Can you work these out from the model? Positions are in its coordinate system, mm. A direction names the side the tool comes from. Round coordinates to 2 decimals unless told otherwise and drop trailing zeros. Loops run counter-clockwise (first coordinate to the right, second up) from the corner with the lowest first, then second, coordinate; pieces in that order, holes last.
from build123d import *

# Parameters (mm, degrees)
ESBO_O1_R                = 6.5
RESSALTO_EXTRUS_O1_DEPTH = 15
RESSALTO_EXTRUS_O2_DEPTH = 35
CORTE_EXTRUS_O1_REACH    = 88.344


with BuildPart() as part:
    # Esboço1 → Ressalto-extrusão1 (new body)
    with BuildSketch(Plane.XY):
        Polygon((-31.616849906, 46.570948478), (-50.373293376, -23.429051522), (-76.616849906, -23.429051522), (-76.616849906, 16.570948478), (-111.616849906, 16.570948478), (-111.616849906, 46.570948478), align=None)
        with Locations((-96.616849906, 31.570948478)):
            Circle(ESBO_O1_R, mode=Mode.SUBTRACT)
    extrude(amount=RESSALTO_EXTRUS_O1_DEPTH)

    # Esboço2 → Ressalto-extrusão2 (add)
    with BuildSketch(Plane(origin=(0, 0, 0), x_dir=(-1, 0, 0), z_dir=(0, 0, -1))):
        Polygon((58.655502819, -23.429051522), (39.899059349, 46.570948478), (31.616849906, 46.570948478), (50.373293376, -23.429051522), align=None)
    extrude(amount=RESSALTO_EXTRUS_O2_DEPTH)

    # Esboço3 → Corte-extrusão1 (cut, up to next)
    with BuildSketch(Plane(origin=(-41.141659675, 11.023874485, 0), x_dir=(0, 0, -1), z_dir=(0.9659258262890673, -0.25881904510252474, 0)), mode=Mode.PRIVATE) as corte_extrus_o1_sk1:
        with BuildLine():
            Line((13, 21.801038988), (13, -16.198961012))
            ThreePointArc((13, -16.198961012), (19, -22.198961012), (25, -16.198961012))
            Line((25, -16.198961012), (25, 21.801038988))
            ThreePointArc((25, 21.801038988), (19, 27.801038988), (13, 21.801038988))
        make_face()
    corte_extrus_o1_tool1 = extrude(corte_extrus_o1_sk1.sketch, amount=-CORTE_EXTRUS_O1_REACH, mode=Mode.PRIVATE) & part.part
    add(corte_extrus_o1_tool1.solids().sort_by_distance((-40.416697, 13.72947, -19))[0], mode=Mode.SUBTRACT)


solid = part.part
(1) Will these pins go through, and if not, where does the flat tip stop? P1, Ø1, axis at x = -55.5, y = 18.5, coming from the -Z side; P2, Ø6, axis at y = -15.5, z = -12.5, coming from the -X side; P3, Ø3, axis at y = 29, z = -4, coming from the -X side.
Worked answers:
P1: stops at z = 0
P2: stops at x = -57.33
P3: stops at x = -45.01
(2) If we section it at A-A, the plane z = -16.5: List the corners of the cut face in (x, y) for me.
Worked answers:
outline: (-58.66, -23.43) - (-50.37, -23.43) - (-46.75, -9.89) - (-54.47, -7.82) - close; (-41.81, 39.42) - (-34.09, 37.35) - (-31.62, 46.57) - (-39.9, 46.57) - close
(3) If we section it at D-D, the plane y = 8.5: List the corners of the cut face in (x, z) for me.
Worked answers:
outline: (-76.62, 0) - (-50.1, 0) - (-50.1, -13) - (-41.82, -13) - (-41.82, 15) - (-76.62, 15) - close; (-50.1, -35) - (-41.82, -35) - (-41.82, -25) - (-50.1, -25) - close
(4) If we mould it in two halves opening along Z, with no side actions, what happens to faces 4 (the flat face through (-44, 14, -25)), 5 (the flat face through (-63, 46.571, 1)), 6 (the flat face through (-43, 12, -35))? For each: released by +Z, released by -Z, zero draft, split by the parting line, or undercut.
Worked answers:
face 4: undercut
face 5: zero draft
face 6: released by -Z
(5) If we section it at B-B, the plane y = 23.5: List the corners of the cut face in (x, z) for me, then the cut area to 3 significant figures.
Worked answers:
outline: (-111.62, 0) - (-46.08, 0) - (-46.08, -13) - (-37.8, -13) - (-37.8, 15) - (-111.62, 15) - close; (-46.08, -35) - (-37.8, -35) - (-37.8, -25) - (-46.08, -25) - close
area: 1,300 mm2
(6) If we section it at C-C, the plane x = -102: List the corners of the cut face in (y, z) for me.
Worked answers:
outline: (16.57, 0) - (27.93, 0) - (27.93, 15) - (16.57, 15) - close; (35.21, 0) - (46.57, 0) - (46.57, 15) - (35.21, 15) - close
(7) If I drill on line 1 (Z direction, x = -47, y = 11.5); line 2 (Y direction, x = -96.5, z = 9); line 3 (Z direction, x = -61.5, y = 24), over which ranges is the centre line in solid material (lowest first)?
Worked answers:
line 1: z = -35 to -25, -13 to 15
line 2: y = 16.57 to 25.07, 38.07 to 46.57
line 3: z = 0 to 15
(8) For faces 1 (the cylindrical face through (-50.696, -9.396, -18.868)), 2 (the flat face through (-94, 16.571, 7)), 3 (the flat face through (-75, 20, 0)), which set-ups out of +Z, -Z, +X, -X, +Y, -Y let a thin tool reach every point of the face, with its end or its side?
Worked answers:
face 1: +X, +Y
face 2: +Z, -Z, -X, -Y
face 3: -Z, -X, +Y
